Source: CAD feature listing. Evaluate the final solid. Frame: model axes, mm. Give positions to 0.01 mm unless a question says otherwise; leave off trailing zeros. Answer as a JSON object with one key per item and string values. Group by question number.
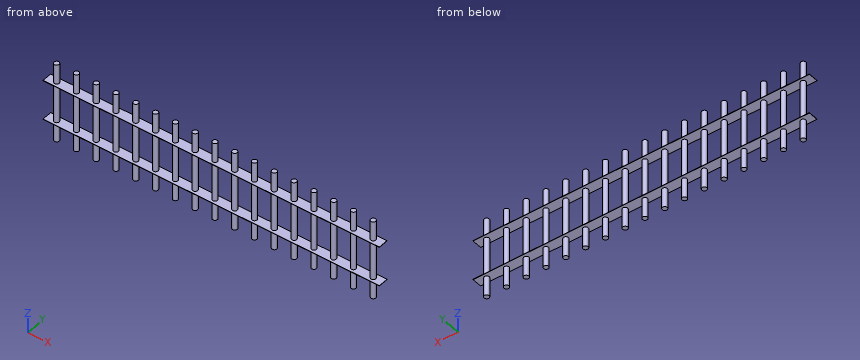
from build123d import *

# Parameters (mm, degrees)
SKETCH1_R              = 3.175
BOSS_EXTRUDE1_DEPTH    = 50.8
BOSS_EXTRUDE1_2_DEPTH  = 50.8
BOSS_EXTRUDE1_3_DEPTH  = 50.8
BOSS_EXTRUDE1_4_DEPTH  = 50.8
BOSS_EXTRUDE1_5_DEPTH  = 50.8
BOSS_EXTRUDE1_6_DEPTH  = 50.8
BOSS_EXTRUDE1_7_DEPTH  = 50.8
BOSS_EXTRUDE1_8_DEPTH  = 50.8
BOSS_EXTRUDE1_9_DEPTH  = 50.8
BOSS_EXTRUDE1_10_DEPTH = 50.8
BOSS_EXTRUDE1_11_DEPTH = 50.8
BOSS_EXTRUDE1_12_DEPTH = 50.8
BOSS_EXTRUDE1_13_DEPTH = 50.8
BOSS_EXTRUDE1_14_DEPTH = 50.8
BOSS_EXTRUDE1_15_DEPTH = 50.8
BOSS_EXTRUDE1_16_DEPTH = 50.8
BOSS_EXTRUDE1_17_DEPTH = 50.8
SKETCH2_W              = 431.8
SKETCH2_H              = 12.7
BOSS_EXTRUDE2_DEPTH    = 0.381


with BuildPart() as part:
    # Sketch1 → Boss-Extrude1 (new body, symmetric)
    with BuildSketch(Plane.XY):
        Circle(SKETCH1_R)
    extrude(amount=BOSS_EXTRUDE1_DEPTH, both=True)



with BuildPart() as body_2:
    # Sketch1 → Boss-Extrude1 2 (new body, symmetric)
    with BuildSketch(Plane.XY):
        with Locations((25.4, 0)):
            Circle(SKETCH1_R)
    extrude(amount=BOSS_EXTRUDE1_2_DEPTH, both=True)


with BuildPart() as body_3:
    # Sketch1 → Boss-Extrude1 3 (new body, symmetric)
    with BuildSketch(Plane.XY):
        with Locations((50.8, 0)):
            Circle(SKETCH1_R)
    extrude(amount=BOSS_EXTRUDE1_3_DEPTH, both=True)


with BuildPart() as body_4:
    # Sketch1 → Boss-Extrude1 4 (new body, symmetric)
    with BuildSketch(Plane.XY):
        with Locations((76.2, 0)):
            Circle(SKETCH1_R)
    extrude(amount=BOSS_EXTRUDE1_4_DEPTH, both=True)


with BuildPart() as body_5:
    # Sketch1 → Boss-Extrude1 5 (new body, symmetric)
    with BuildSketch(Plane.XY):
        with Locations((101.6, 0)):
            Circle(SKETCH1_R)
    extrude(amount=BOSS_EXTRUDE1_5_DEPTH, both=True)


with BuildPart() as body_6:
    # Sketch1 → Boss-Extrude1 6 (new body, symmetric)
    with BuildSketch(Plane.XY):
        with Locations((127, 0)):
            Circle(SKETCH1_R)
    extrude(amount=BOSS_EXTRUDE1_6_DEPTH, both=True)


with BuildPart() as body_7:
    # Sketch1 → Boss-Extrude1 7 (new body, symmetric)
    with BuildSketch(Plane.XY):
        with Locations((152.4, 0)):
            Circle(SKETCH1_R)
    extrude(amount=BOSS_EXTRUDE1_7_DEPTH, both=True)


with BuildPart() as body_8:
    # Sketch1 → Boss-Extrude1 8 (new body, symmetric)
    with BuildSketch(Plane.XY):
        with Locations((177.8, 0)):
            Circle(SKETCH1_R)
    extrude(amount=BOSS_EXTRUDE1_8_DEPTH, both=True)


with BuildPart() as body_9:
    # Sketch1 → Boss-Extrude1 9 (new body, symmetric)
    with BuildSketch(Plane.XY):
        with Locations((203.2, 0)):
            Circle(SKETCH1_R)
    extrude(amount=BOSS_EXTRUDE1_9_DEPTH, both=True)


with BuildPart() as body_10:
    # Sketch1 → Boss-Extrude1 10 (new body, symmetric)
    with BuildSketch(Plane.XY):
        with Locations((228.6, 0)):
            Circle(SKETCH1_R)
    extrude(amount=BOSS_EXTRUDE1_10_DEPTH, both=True)


with BuildPart() as body_11:
    # Sketch1 → Boss-Extrude1 11 (new body, symmetric)
    with BuildSketch(Plane.XY):
        with Locations((254, 0)):
            Circle(SKETCH1_R)
    extrude(amount=BOSS_EXTRUDE1_11_DEPTH, both=True)


with BuildPart() as body_12:
    # Sketch1 → Boss-Extrude1 12 (new body, symmetric)
    with BuildSketch(Plane.XY):
        with Locations((279.4, 0)):
            Circle(SKETCH1_R)
    extrude(amount=BOSS_EXTRUDE1_12_DEPTH, both=True)


with BuildPart() as body_13:
    # Sketch1 → Boss-Extrude1 13 (new body, symmetric)
    with BuildSketch(Plane.XY):
        with Locations((304.8, 0)):
            Circle(SKETCH1_R)
    extrude(amount=BOSS_EXTRUDE1_13_DEPTH, both=True)


with BuildPart() as body_14:
    # Sketch1 → Boss-Extrude1 14 (new body, symmetric)
    with BuildSketch(Plane.XY):
        with Locations((330.2, 0)):
            Circle(SKETCH1_R)
    extrude(amount=BOSS_EXTRUDE1_14_DEPTH, both=True)


with BuildPart() as body_15:
    # Sketch1 → Boss-Extrude1 15 (new body, symmetric)
    with BuildSketch(Plane.XY):
        with Locations((355.6, 0)):
            Circle(SKETCH1_R)
    extrude(amount=BOSS_EXTRUDE1_15_DEPTH, both=True)


with BuildPart() as body_16:
    # Sketch1 → Boss-Extrude1 16 (new body, symmetric)
    with BuildSketch(Plane.XY):
        with Locations((381, 0)):
            Circle(SKETCH1_R)
    extrude(amount=BOSS_EXTRUDE1_16_DEPTH, both=True)


with BuildPart() as body_17:
    # Sketch1 → Boss-Extrude1 17 (new body, symmetric)
    with BuildSketch(Plane.XY):
        with Locations((406.4, 0)):
            Circle(SKETCH1_R)
    extrude(amount=BOSS_EXTRUDE1_17_DEPTH, both=True)


with BuildPart() as part_1:
    add(part.part)

    add(body_2.part)  # Boss-Extrude2 merges body 2

    add(body_3.part)  # Boss-Extrude2 merges body 3

    add(body_4.part)  # Boss-Extrude2 merges body 4

    add(body_5.part)  # Boss-Extrude2 merges body 5

    add(body_6.part)  # Boss-Extrude2 merges body 6

    add(body_7.part)  # Boss-Extrude2 merges body 7

    add(body_8.part)  # Boss-Extrude2 merges body 8

    add(body_9.part)  # Boss-Extrude2 merges body 9

    add(body_10.part)  # Boss-Extrude2 merges body 10

    add(body_11.part)  # Boss-Extrude2 merges body 11

    add(body_12.part)  # Boss-Extrude2 merges body 12

    add(body_13.part)  # Boss-Extrude2 merges body 13

    add(body_14.part)  # Boss-Extrude2 merges body 14

    add(body_15.part)  # Boss-Extrude2 merges body 15

    add(body_16.part)  # Boss-Extrude2 merges body 16

    add(body_17.part)  # Boss-Extrude2 merges body 17
    # Sketch2 → Boss-Extrude2 (add)
    with BuildSketch(Plane.XY.offset(25.4)):
        with Locations((203.2, 0)):
            Rectangle(SKETCH2_W, SKETCH2_H)
    boss_extrude2 = extrude(amount=BOSS_EXTRUDE2_DEPTH)

    # Mirror1: Boss-Extrude2 across plane
    add(boss_extrude2.mirror(Plane.XY))


solid = part_1.part
Q1. Ray query, probe 1 along Z at (x, y) = (361, -3.5); probe 2 along Y at (x, z) = (102, -14); probe 3 along Y at (x, z) = (25.5, 9). Return the intervals inside material, ascending. Write a range as [from, to].
Q2. First-contact query: pin 1 Ø2 at (y, z) = (-3, 12.5) entering from +X; pin 2 Ø4 at (x, y) = (209, 0.5) entering from -Z; pin 3 Ø5 at (x, z) = (257.5, 0) entering from +Y; pin 4 Ø8 at (x, z) = (170, -14.5) entering from +Y. Flat tips, straight axial feed; report the tip coordinate or a pass-through.
Q3. Section A-A on z = -39.5. State how many separate pieces and enclosed holes the cut face has, then the cut area to 3 significant figures.
Taken from the geometry:
{
 "1": {"probe 1": "z = [-25.78, -25.4], [25.4, 25.78]", "probe 2": "y = [-3.15, 3.15]", "probe 3": "y = [-3.17, 3.17]"},
 "2": {"pin 1": "stops at x = 408.87", "pin 2": "stops at z = -25.78", "pin 3": "stops at y = 3.01", "pin 4": "passes through"},
 "3": {"separate pieces": "17", "enclosed holes": "0", "area": "538 mm²"}
}
